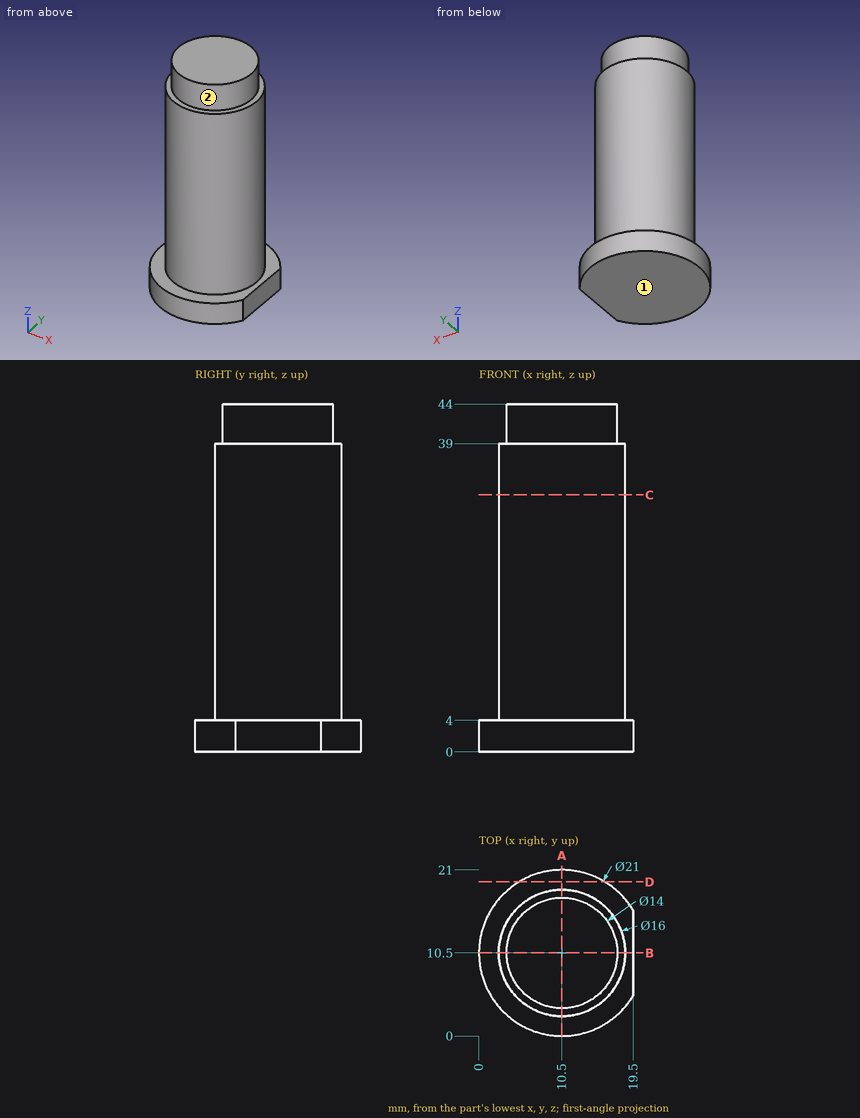
The figure shows three views and two pictorial views of one solid part (mm, origin at its lowest corner). Answer the questions. A direction names the side the tool comes from. Give positions to 0.01 mm unless a question says otherwise; leave off trailing zeros. Loops run counter-clockwise (first coordinate to the right, second up) from the corner with the lowest first, then second, coordinate; pieces in that order, holes last. Notation, with made-up numbers: (6, 19.5) -> (14, 19.5) arc R37 ccw to (14, 56.5) -> close; hole circle Ø4 at (-4, 53.5). An arc over 180 degrees is marked (long way). Use a Markdown table: item, result. Add a question column.
1. Flat-ended cylindrical pins translate along their axes: pin 1 Ø6 at (x, z) = (5.5, 9) entering from -Y; pin 2 Ø10 at (y, z) = (11, 10) entering from -X; pin 3 Ø10 at (x, z) = (3.5, 11) entering from +Y; pin 4 Ø4 at (x, y) = (6, 3) entering from +Z. Find the tip coordinate at first contact, or state that the pin passes through.
2. Section D-D on y = 19.5 is taken. Determine the outline of the cut face in (x, z), and give its area (3 significant figures).
3. Section C-C on z = 32.5 is taken. Determine the outline of the cut face in (x, y).
4. Section A-A on x = 10.5 is taken. Determine the outline of the cut face in (y, z), and give its area (3 significant figures).
5. For the marked faces 1 and 2, determine the directions among +Z, -Z, +X, -X, +Y, -Y from which every point of the face is accessible in a straight line to the end or side of a thin tool.
6. Find the intervals of material crossed by probe 1 along Z at (x, y) = (16, 15.5); probe 2 along Z at (x, y) = (14, 18.25); probe 3 along Y at (x, z) = (10.75, 14), in increasing order.
7. Section B-B on y = 10.5 is taken. Determine the outline of the cut face in (x, z), and give its area (3 significant figures).
Results below:
| question | item | result |
|---|---|---|
| 1 | pin 1 | stops at y = 2.75 |
| 1 | pin 2 | stops at x = 2.5 |
| 1 | pin 3 | stops at y = 18.25 |
| 1 | pin 4 | stops at z = 44 |
| 2 | outline | (5.09, 0) -> (15.91, 0) -> (15.91, 4) -> (5.09, 4) -> close |
| 2 | area | 43.3 mm^2 |
| 3 | outline | circle Ø16 at (10.5, 10.5) |
| 4 | outline | (0, 0) -> (21, 0) -> (21, 4) -> (18.5, 4) -> (18.5, 39) -> (17.5, 39) -> (17.5, 44) -> (3.5, 44) -> (3.5, 39) -> (2.5, 39) -> (2.5, 4) -> (0, 4) -> close |
| 4 | area | 714 mm^2 |
| 5 | face 1 | -Z, +X, -X, +Y, -Y |
| 5 | face 2 | +Z |
| 6 | probe 1 | z = 0 to 39 |
| 6 | probe 2 | z = 0 to 4 |
| 6 | probe 3 | y = 2.5 to 18.5 |
| 7 | outline | (0, 0) -> (19.5, 0) -> (19.5, 4) -> (18.5, 4) -> (18.5, 39) -> (17.5, 39) -> (17.5, 44) -> (3.5, 44) -> (3.5, 39) -> (2.5, 39) -> (2.5, 4) -> (0, 4) -> close |
| 7 | area | 708 mm^2 |
